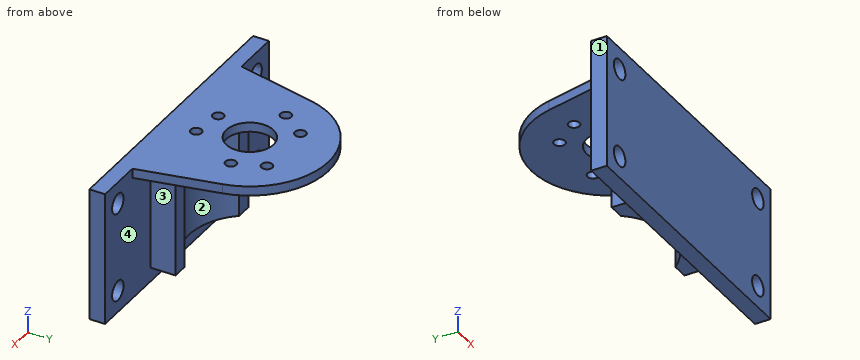
```python
from build123d import *

# Parameters (mm, degrees)
SKETCH3_W           = 90
SKETCH3_H           = 42.5
SKETCH3_R           = 3.15
BOSS_EXTRUDE1_DEPTH = 5
SKETCH4_R           = 1.75
SKETCH4_R_2         = 7.5
BOSS_EXTRUDE2_DEPTH = 3
SKETCH5_W           = 5
SKETCH5_H           = 7.935071488
BOSS_EXTRUDE3_DEPTH = 35


with BuildPart() as part:
    # Sketch3 → Boss-Extrude1 (new body)
    with BuildSketch(Plane(origin=(0, 0, 0), x_dir=(1, 0, 0), z_dir=(0, 1, 0))):
        Rectangle(SKETCH3_W, SKETCH3_H)
        with Locations(Location((-38, 14.25, 0), (0, 0, 270))):
            Circle(SKETCH3_R, mode=Mode.SUBTRACT)
        with Locations(Location((38, 14.25, 0), (0, 0, 90))):
            Circle(SKETCH3_R, mode=Mode.SUBTRACT)
        with Locations(Location((38, -14.25, 0), (0, 0, 270))):
            Circle(SKETCH3_R, mode=Mode.SUBTRACT)
        with Locations(Location((-38, -14.25, 0), (0, 0, 90))):
            Circle(SKETCH3_R, mode=Mode.SUBTRACT)
    extrude(amount=BOSS_EXTRUDE1_DEPTH)

    # Sketch4 → Boss-Extrude2 (add)
    with BuildSketch(Plane.XY.offset(21.25)):
        with BuildLine():
            Line((-30, 5), (30, 5))
            Line((30, 5), (24.415677736, 30.373516604))
            ThreePointArc((24.415677736, 30.373516604), (0, 50), (-24.415677736, 30.373516604))
            Line((-24.415677736, 30.373516604), (-30, 5))
        make_face()
        with Locations((10.21923709, 36.347341968)):
            Circle(SKETCH4_R, mode=Mode.SUBTRACT)
        with Locations((-5.067303705, 12.010919994)):
            Circle(SKETCH4_R, mode=Mode.SUBTRACT)
        with Locations((4.749376983, 10.674714152)):
            Circle(SKETCH4_R, mode=Mode.SUBTRACT)
        with Locations((0, 25)):
            Circle(SKETCH4_R_2, mode=Mode.SUBTRACT)
        with Locations((13.990382911, 27.080076467)):
            Circle(SKETCH4_R, mode=Mode.SUBTRACT)
        with Locations((-14.667309102, 27.992284383)):
            Circle(SKETCH4_R, mode=Mode.SUBTRACT)
        with Locations((-8.654917128, 36.087456884)):
            Circle(SKETCH4_R, mode=Mode.SUBTRACT)
    extrude(amount=-BOSS_EXTRUDE2_DEPTH)

    # Sketch5 → Boss-Extrude3 (add)
    with BuildSketch(Plane(origin=(0, 0, 18.25), x_dir=(-1, 0, 0), z_dir=(0, 0, -1))):
        with BuildLine():
            ThreePointArc((15, 12.935071488), (0, 5.75), (-15, 12.935071488))
            Line((-15, 12.935071488), (-15, 5))
            Line((-15, 5), (15, 5))
            Line((15, 5), (15, 12.935071488))
        make_face()
        with Locations((-17.5, 8.967535744)):
            Rectangle(SKETCH5_W, SKETCH5_H)
        with Locations((17.5, 8.967535744)):
            Rectangle(SKETCH5_W, SKETCH5_H)
    extrude(amount=BOSS_EXTRUDE3_DEPTH)


solid = part.part
```
The listing builds one solid part. Answer for the finished solid, in the listing's coordinates (mm). Face numbers are marked on the shaded views. Round coordinates to 2 decimals unless told otherwise and drop trailing zeros. Loops run counter-clockwise (first coordinate to the right, second up) from the corner with the lowest first, then second, coordinate; pieces in that order, holes last.
Q1. Section D-D, the plane z = 7 is taken. Determine the outline of the cut face in (x, y), then the cut area to 3 significant figures.
Q2. Section A-A, the plane z = 14.25 is taken. Determine the outline of the cut face in (x, y), then the cut area to 3 significant figures.
Q3. For a pull along X with two mould halves and no side action, classify the marked faces 1, 2, 3 and 4 as released by +X, released by -X, zero draft, split by the parting line, or undercut.
Q4. Find the intervals of material crossed by line 1 (X direction, y = 2.3, z = -14.25); line 2 (Y direction, x = -3.5, z = 18.5); line 3 (Z direction, x = 6.5, y = 42), in increasing order.
Q5. Section C-C, the plane x = 0 is taken. Determine the outline of the cut face in (y, z).
Q6. Given pin 1 Ø6 at (x, y) = (-5, 35) entering from -Z; pin 2 Ø4 at (x, y) = (4, 8) entering from -Z; pin 3 Ø1.5 at (x, z) = (1, 7) entering from +Y, each flat-ended and moving along its own axis, determine where each tip first touches the part or whether it passes through.
Q7. Section B-B, the plane x = -38 is taken. Determine the outline of the cut face in (y, z), then the cut area to 4 significant figures.
Completed:
1. outline: (-45, 0) - (45, 0) - (45, 5) - (20, 5) - (20, 12.94) - (15, 12.94) arc R19.25 cw to (-15, 12.94) - (-20, 12.94) - (-20, 5) - (-45, 5) - close
1. area: 617 mm2
2. outline: (-45, 0) - (-41.15, 0) - (-41.15, 5) - (-45, 5) - close; (-34.85, 0) - (34.85, 0) - (34.85, 5) - (20, 5) - (20, 12.94) - (15, 12.94) arc R19.25 cw to (-15, 12.94) - (-20, 12.94) - (-20, 5) - (-34.85, 5) - close; (41.15, 0) - (45, 0) - (45, 5) - (41.15, 5) - close
2. area: 554 mm2
3. face 1: released by -X
3. face 2: undercut
3. face 3: released by +X
3. face 4: zero draft
4. line 1: x = -45 to -41.15, -34.85 to 34.85, 41.15 to 45
4. line 2: y = 0 to 11.23, 12.79 to 18.37, 31.63 to 49.75
4. line 3: z = 18.25 to 21.25
5. outline: (0, -21.25) - (5, -21.25) - (5, -16.75) - (5.75, -16.75) - (5.75, 18.25) - (17.5, 18.25) - (17.5, 21.25) - (0, 21.25) - close; (32.5, 18.25) - (50, 18.25) - (50, 21.25) - (32.5, 21.25) - close
6. pin 1: stops at z = 18.25
6. pin 2: stops at z = -16.75
6. pin 3: stops at y = 5.83
7. outline: (0, -21.25) - (5, -21.25) - (5, -17.4) - (0, -17.4) - close; (0, -11.1) - (5, -11.1) - (5, 11.1) - (0, 11.1) - close; (0, 17.4) - (5, 17.4) - (5, 21.25) - (0, 21.25) - close
7. area: 149.5 mm2
